Source: CAD feature listing. Evaluate the final solid. Frame: model axes, mm. Face numbers are marked on the shaded views. A direction names the side the tool comes from. Round coordinates to 2 decimals unless told otherwise and drop trailing zeros. Order: outer loops, then holes, each group sorted by start corner. A loop starts at its lowest first (then second) coordinate and runs counter-clockwise, first axis right, second up. Notation, with made-up numbers: M 85,70 L 107,70 A5 cw 107,79 Z; hole C 71,80 d7. An arc over 180 degrees is marked long. Answer in a Markdown table with one row per item. Add a question column.
```python
from build123d import *

# Parameters (mm, degrees)
BOSS_EXTRUDE1_DEPTH = 14.2
SKETCH2_R           = 2
CUT_EXTRUDE1_DEPTH  = 3


with BuildPart() as part:
    # Sketch1 → Boss-Extrude1 (new body)
    with BuildSketch(Plane.XY):
        with BuildLine():
            Line((0, 0), (12, 0))
            Line((12, 0), (14, 0))
            ThreePointArc((14, 0), (14.707106781, 0.292893219), (15, 1))
            Line((15, 1), (15, 12.7))
            Line((15, 12.7), (23.7, 12.7))
            ThreePointArc((23.7, 12.7), (24.407106781, 12.992893219), (24.7, 13.7))
            Line((24.7, 13.7), (24.7, 23))
            Line((24.7, 23), (26.8, 23))
            Line((26.8, 23), (26.8, 13.7))
            ThreePointArc((26.8, 13.7), (27.092893219, 12.992893219), (27.8, 12.7))
            Line((27.8, 12.7), (33.1, 12.7))
            Line((33.1, 12.7), (33.1, 1))
            ThreePointArc((33.1, 1), (33.392893219, 0.292893219), (34.1, 0))
            Line((34.1, 0), (48.1, 0))
            Line((48.1, 0), (48.1, 2))
            ThreePointArc((48.1, 2), (47.807106781, 2.707106781), (47.1, 3))
            Line((47.1, 3), (37.1, 3))
            ThreePointArc((37.1, 3), (36.392893219, 3.292893219), (36.1, 4))
            Line((36.1, 4), (36.1, 14.7))
            ThreePointArc((36.1, 14.7), (35.807106781, 15.407106781), (35.1, 15.7))
            Line((35.1, 15.7), (30.8, 15.7))
            ThreePointArc((30.8, 15.7), (30.092893219, 15.992893219), (29.8, 16.7))
            Line((29.8, 16.7), (29.8, 25))
            ThreePointArc((29.8, 25), (29.507106781, 25.707106781), (28.8, 26))
            Line((28.8, 26), (22.7, 26))
            ThreePointArc((22.7, 26), (21.992893219, 25.707106781), (21.7, 25))
            Line((21.7, 25), (21.7, 16.7))
            ThreePointArc((21.7, 16.7), (21.407106781, 15.992893219), (20.7, 15.7))
            Line((20.7, 15.7), (13, 15.7))
            ThreePointArc((13, 15.7), (12.292893219, 15.407106781), (12, 14.7))
            Line((12, 14.7), (12, 4))
            ThreePointArc((12, 4), (11.707106781, 3.292893219), (11, 3))
            Line((11, 3), (1, 3))
            ThreePointArc((1, 3), (0.292893219, 2.707106781), (0, 2))
            Line((0, 2), (0, 0))
        make_face()
    extrude(amount=-BOSS_EXTRUDE1_DEPTH)

    # Sketch2 → Cut-Extrude1 (cut)
    with BuildSketch(Plane(origin=(0, 0, 0), x_dir=(1, 0, 0), z_dir=(0, 1, 0))):
        with Locations(Location((42.1, 7.1, 0), (0, 0, 180))):  # turned: the seam where the file's is
            Circle(SKETCH2_R)
        with Locations(Location((6, 7.1, 0), (0, 0, 180))):  # turned: the seam where the file's is
            Circle(SKETCH2_R)
    extrude(amount=CUT_EXTRUDE1_DEPTH, mode=Mode.SUBTRACT)


solid = part.part
```
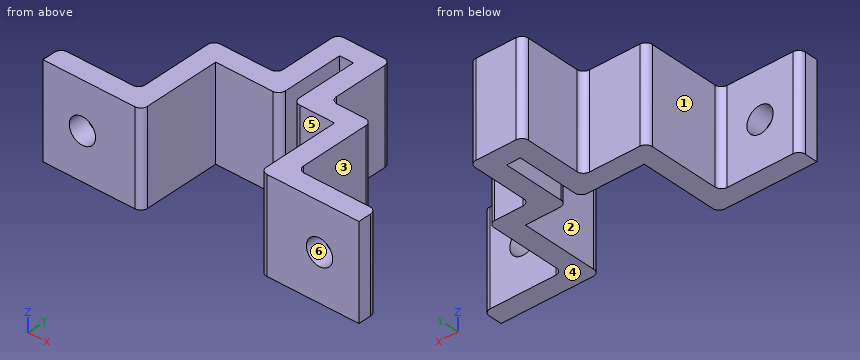
(1) Draft query along Z for the marked faces 4, 5 and 6. Return one class per face: +Z half, -Z half, draft (parallel to the pull), parting line (faces both ways), or undercut.
(2) Cut plane A-A (x = 42.1). Return loops of the section in (y, z).
(3) Cut plane C-C (z = -7.1). Count the separate pieces of the cut face and the enclosed holes in it, and give its area (3 significant figures).
(4) Access query for the marked faces 1, 2 and 3. Directions: +Z, -Z, +X, -X, +Y, -Y. A direction counts if a zero-diameter tool reaches every point of the face in a straight line with its end or side. Return the directions, or none.
(5) Cut plane B-B (y = 10). Return loops of the section in (x, z).
(6) Line query: line 1 (X direction, y = 17.75, z = -3.25); line 2 (Z direction, x = 6, y = 1.7); line 3 (X direction, y = 7.75, z = -9). Output: solid intervals per line, ascending. Write a range as from..to.
(7) Pin query (flat end, axial travel): pin 1 (6 mm diameter, centred on x = 15.5, y = 10, fed in from -Z); pin 2 (5 mm diameter, centred on x = 17, y = 19.5, fed in from +Z); pin 3 (3 mm diameter, centred on x = 27, z = -3.5, fed in from -Y); pin 4 (2.5 mm diameter, centred on x = 25.5, z = -9.5, fed in from -Y). Return the tip coordinate at first contact, or that it passes through.
Answer list:
| question | item | result |
|---|---|---|
| 1 | face 4 | -Z half |
| 1 | face 5 | draft |
| 1 | face 6 | undercut |
| 2 | outline | M 0,-14.2 L 3,-14.2 L 3,-9.1 L 0,-9.1 Z; M 0,-5.1 L 3,-5.1 L 3,0 L 0,0 Z |
| 3 | separate pieces | 3 |
| 3 | enclosed holes | 0 |
| 3 | area | 257 mm² |
| 4 | face 1 | +Z, -Z, -X, +Y |
| 4 | face 2 | +Z, -Z, -Y |
| 4 | face 3 | +Z, -Z, +X, +Y |
| 5 | outline | M 12,-14.2 L 15,-14.2 L 15,0 L 12,0 Z; M 33.1,-14.2 L 36.1,-14.2 L 36.1,0 L 33.1,0 Z |
| 6 | line 1 | 21.7..24.7, 26.8..29.8 |
| 6 | line 2 | -14.2..-9.1, -5.1..0 |
| 6 | line 3 | 12..15, 33.1..36.1 |
| 7 | pin 1 | z = -14.2 |
| 7 | pin 2 | through |
| 7 | pin 3 | y = 12.7 |
| 7 | pin 4 | y = 12.86 |
